from build123d import *

# Parameters (mm, degrees)
F0_R      = 26
F1_DEPTH  = 44
F2_T      = -3
F4_DEPTH  = 5
F5_W      = 13
F5_H      = 24
F6_DEPTH  = 25
F7_R      = 0.9
F8_DEPTH  = 44.001
F9_R      = 5.5
F10_DEPTH = 2
F11_R     = 5


with BuildPart() as f1:
    # F0 (on Front) → F1 (new body)
    with BuildSketch(Plane.XZ):
        Circle(F0_R)
    extrude(amount=F1_DEPTH)

    # F2
    f2_openings = [f1.faces().sort_by_distance(p)[0] for p in [
        (0, 0, 0),
    ]]
    offset(amount=F2_T, openings=f2_openings)

    # F3 (on Front) → F4 (join)
    with BuildSketch(Plane.XZ):
        with BuildLine():
            ThreePointArc((-24.8986899768, -7.4870045706), (-25.9999991145, 0.0067856521), (-24.894778569, 7.5))
            Line((-24.894778569, 7.5), (-29.5586808862, 7.5))
            Line((-29.5586808862, 7.5), (-29.5586808862, 7.4870045706))
            ThreePointArc((-29.5586808862, 7.4870045706), (-37.5, 0), (-29.5586808862, -7.4870045706))
            Line((-29.5586808862, -7.4870045706), (-24.8986899768, -7.4870045706))
        make_face()
        with BuildLine():
            Line((7.5, 24.894778569), (7.5, 30))
            ThreePointArc((7.5, 30), (0, 37.5), (-7.5, 30))
            Line((-7.5, 30), (-7.5, 24.894778569))
            ThreePointArc((-7.5, 24.894778569), (0, 26), (7.5, 24.894778569))
        make_face()
        with BuildLine():
            Line((-7.5, -24.894778569), (-7.5, -30))
            ThreePointArc((-7.5, -30), (0, -37.5), (7.5, -30))
            Line((7.5, -30), (7.5, -24.894778569))
            ThreePointArc((7.5, -24.894778569), (0, -26), (-7.5, -24.894778569))
        make_face()
        with BuildLine():
            Line((30.4413191138, -7.4870045706), (29.5586808862, -7.4870045706))
            ThreePointArc((29.5586808862, -7.4870045706), (30, -7.5), (30.4413191138, -7.4870045706))
        make_face()
        with BuildLine():
            Line((24.8986899768, -7.4870045706), (29.5586808862, -7.4870045706))
            Line((29.5586808862, -7.4870045706), (30.4413191138, -7.4870045706))
            ThreePointArc((30.4413191138, -7.4870045706), (37.4967504387, 0.2207552046), (30, 7.5))
            Line((30, 7.5), (24.894778569, 7.5))
            ThreePointArc((24.894778569, 7.5), (25.9999991145, 0.0067856521), (24.8986899768, -7.4870045706))
        make_face()
    extrude(amount=F4_DEPTH)

    # F5 (on face) → F6 (cut)
    with BuildSketch(Plane.XZ.offset(44)):
        with Locations((0, 5)):
            Rectangle(F5_W, F5_H)
    extrude(amount=-F6_DEPTH, mode=Mode.SUBTRACT)

    # F7 (on face) → F8 (cut, through all)
    with BuildSketch(Plane.XZ.offset(44)):
        with Locations((0, -8.7)):
            Circle(F7_R)
        with Locations((0, 19.1)):
            Circle(F7_R)
    extrude(amount=-F8_DEPTH, mode=Mode.SUBTRACT)

    # F9 (on face) → F10 (cut)
    with BuildSketch(Plane(origin=(0, 0, 0), x_dir=(-1, 0, 0), z_dir=(0, 1, 0))):
        with Locations((-30, 0)):
            Circle(F9_R)
        with Locations((0, 30)):
            Circle(F9_R)
        with Locations((30, 0)):
            Circle(F9_R)
        with Locations((0, -30)):
            Circle(F9_R)
    extrude(amount=-F10_DEPTH, mode=Mode.SUBTRACT)

    # F11
    f11_edges = [f1.edges().sort_by_distance(p)[0] for p in [
        (24.89869, -2.5, -7.487005),
        (7.5, -2.5, -24.894779),
        (-7.5, -2.5, -24.894779),
        (-24.89869, -2.5, -7.487005),
        (-24.894779, -2.5, 7.5),
        (-7.5, -2.5, 24.894779),
        (7.5, -2.5, 24.894779),
        (24.894779, -2.5, 7.5),
    ]]
    fillet(f11_edges, radius=F11_R)


solid = f1.part
Model file for the job. Use its own axes, mm. A direction names the side the tool comes from. Give positions to 0.01 mm unless a question says otherwise; leave off trailing zeros. Loops run counter-clockwise (first coordinate to the right, second up) from the corner with the lowest first, then second, coordinate; pieces in that order, holes last.
1) Saw through at A-A (z = 0). Write the cut outline in (x, y).
2) Wall check: line 1 (Z direction, x = 0, y = -0.75); line 2 (Z direction, x = 0, y = -43); line 3 (Z direction, x = -30, y = -0.9). Give the ranges that are in metal, low to high.
3) Saw through at C-C (x = 4). Write the cut outline in (y, z).
4) Flat gauge pins, fed straight in: pin 1 Ø2.5 at (y, z) = (-43, 1.5) entering from -X; pin 2 Ø0.5 at (y, z) = (-3, 29.5) entering from +X; pin 3 Ø4 at (x, z) = (-5, -31.5) entering from -Y. Where does each tip first touch, or does it go through?
5) Saw through at D-D (x = 16). Write the cut outline in (y, z).
6) Tool access for faces 1 (the flat face through (-30, -2, 0)), 2 (the flat face through (6.5, -43, 5)), 3 (the cylindrical face through (8.334, -2.535, 25.603)): list every direction of +Z, -Z, +X, -X, +Y, -Y with a clear straight run to the whole face (end or side of a thin tool).
7) Pull direction Z, two halves, no side cores. Call faces 4 (the cylindrical face through (-37.5, -2.46, 0.17)), 5 (the flat face through (0, -2, 30)), 6 (the cylindrical face through (-8.334, -2.535, 25.603)), 7 (the flat face through (0, -44, -11)): +Z half, -Z half, draft (parallel to the pull), parting line (faces both ways), or undercut.
Answer block:
1. outline: (-37.5, -5) - (-26, -5) - (-26, -44) - (-6.5, -44) - (-6.5, -41) - (-23, -41) - (-23, 0) - (-24.5, 0) - (-24.5, -2) - (-35.5, -2) - (-35.5, 0) - (-37.5, 0) - close; (6.5, -44) - (26, -44) - (26, -5) - (37.5, -5) - (37.5, 0) - (35.5, 0) - (35.5, -2) - (24.5, -2) - (24.5, 0) - (23, 0) - (23, -41) - (6.5, -41) - close
2. line 1: z = -37.5 to -35.5, -24.5 to -23, 23 to 24.5, 35.5 to 37.5
2. line 2: z = -26 to -9.6, -7.8 to -7, 17 to 18.2, 20 to 26
2. line 3: z = -7.5 to -5.5, 5.5 to 7.5
3. outline: (-44, -25.69) - (-5, -25.69) - (-5, -36.34) - (0, -36.34) - (0, -33.77) - (-2, -33.77) - (-2, -26.23) - (0, -26.23) - (0, -22.65) - (-41, -22.65) - (-41, -7) - (-44, -7) - close; (-44, 17) - (-41, 17) - (-41, 22.65) - (0, 22.65) - (0, 26.23) - (-2, 26.23) - (-2, 33.77) - (0, 33.77) - (0, 36.34) - (-5, 36.34) - (-5, 25.69) - (-44, 25.69) - close
4. pin 1: stops at x = -26
4. pin 2: stops at x = 7.5
4. pin 3: stops at y = -5
5. outline: (-44, -20.49) - (0, -20.49) - (0, -16.52) - (-41, -16.52) - (-41, 16.52) - (0, 16.52) - (0, 20.49) - (-44, 20.49) - close
6. face 1: +Y
6. face 2: +Y, -Y
6. face 3: +Z, +X, +Y, -Y
7. face 4: parting line
7. face 5: undercut
7. face 6: +Z half
7. face 7: draft
